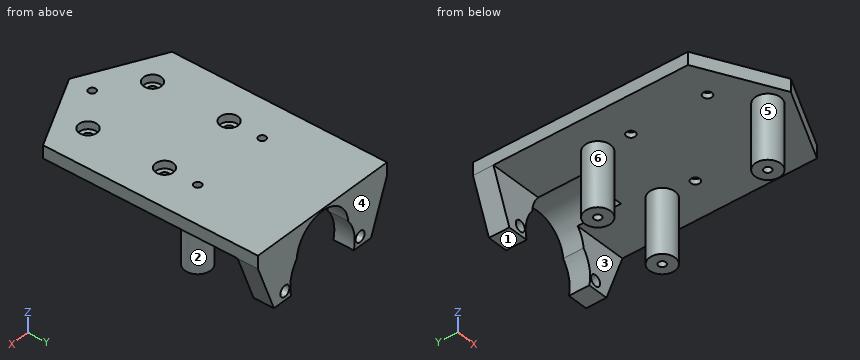
Autodesk Inventor part; units mm, degrees
ref_plane "YZ Plane" through (0, 0, 0) normal (1, 0, 0) x (0, 1, 0)
ref_plane "XZ Plane" through (0, 0, 0) normal (0, 1, 0) x (-1, 0, 0)
ref_plane "XY Plane" through (0, 0, 0) normal (0, 0, 1) x (1, 0, 0)
ref_plane "Work Plane1" through (0, 0, 0) normal (0, 0, 1) x (1, 0, 0)
sketch "Sketch1" plane through (0, 0, 0) normal (0, 0, 1) x (1, 0, 0)
  circle A0 centre (-15, -15) radius 1.5
  circle A1 centre (15, 15) radius 1.5
  circle A2 centre (15, -15) radius 1.5
  circle A3 centre (-15, 15) radius 1.5
  line L0 (30, 20) -> (-30, 20) construction
  line L1 (-30, 20) -> (-30, -20)
  line L2 (-30, -20) -> (30, -20)
  line L3 (30, -20) -> (30, 20)
  line L4 (30, 20) -> (-30, 20)
  line L5 (-30, 20) -> (-30, 64.25)
  line L6 (-30, 64.25) -> (30, 64.25)
  line L7 (30, 64.25) -> (30, 20)
  line L8 (13.5554, 64.25) -> (17.5, 64.25)
  line L9 (-30, -20) -> (0, -35)
  line L10 (0, -35) -> (30, -20)
  line L11 (-0.0001, -26) -> (-15, 28) construction
  line L12 (-15, 28) -> (15, 28) construction
  line L13 (15, 28) -> (-0.0001, -26) construction
  circle A4 centre (-15, 28) radius 1.45
  circle A5 centre (15, 28) radius 1.45
  circle A6 centre (0, -26.0002) radius 1.45
  line L14 (-30, -20) -> (30, -20)
  line L15 (30, -20) -> (30, 20)
  line L16 (30, 20) -> (-30, 20)
  line L17 (-30, 20) -> (-30, -20)
  point P0 (0, 0)
  dimension "d19" = 15
  dimension "d20" = 2.9
  dimension "d21" = 2.9
  dimension "d22" = 2.9
  dimension "d23" = 30
  dimension "d24" = 28
  dimension "d30" = 0
  dimension "d31" = 26
extrude "Extrusion1" add sketch "Sketch1" along normal blind 5 contours A0 | A1 | A2 | A3 | L4 L3 L2 L1 | L5 L6 L7 L4 | L2 L10 L9
sketch "Sketch2" plane through (0, 0, 5) normal (0, 0, 1) x (1, 0, 0)
  circle A0 centre (15, 15) radius 1.5
  circle A1 centre (15, -15) radius 1.5
  circle A2 centre (-20, 13) radius 1.5
  circle A3 centre (-20, -13) radius 1.5
  circle A4 centre (-15, -15) radius 1.5
  circle A5 centre (-15, 15) radius 1.5
  point P0 (0, 0)
hole "Hole1" at (15, 15, 5) at (15, -15, 5) at (-15, -15, 5) at (-15, 15, 5) direction (0, 0, -1) diameter 3.5 depth 8 tip angle 118 counterbore diameter 7 counterbore depth 3
sketch "Sketch3" plane through (-30, 64.25, 0) normal (0, 1, 0) x (1, 0, 0)
  circle A0 centre (12.5, 15.7367) radius 2.1
  circle A1 centre (47.5, 15.7367) radius 2.1
  arc A2 (16, 15.7367) -> (44, 15.7367) centre (30, 15.7367) ccw
  circle A3 centre (30, 15.7367) radius 15
  line L0 (12.5, 19.2367) -> (16.4446, 19.2367)
  line L1 (43.5554, 19.2367) -> (47.5, 19.2367)
  line L2 (15.414, 19.2367) -> (7.414, 19.2367)
  line L3 (0, 0) -> (60, 0)
  line L4 (7.414, 19.2367) -> (0, 0)
  line L5 (0, 0) -> (60, 0)
  line L6 (44.586, 19.2367) -> (52.586, 19.2367)
  line L7 (52.586, 19.2367) -> (60, 0)
  circle A4 centre (12.5, 15.7367) radius 1.45
  circle A5 centre (47.5, 15.7367) radius 1.45
  point P0 (30, 0)
  dimension "d9" = 30
  dimension "d10" = 8
  dimension "d11" = 8
  dimension "d12" = 2.9
  dimension "d13" = 2.9
extrude "Extrusion2" add sketch "Sketch3" against normal blind 8 contours A3 L1 L6 L7 L3 L4 L2 L0
sketch "Sketch4" plane through (-30, 64.25, 5) normal (0, 1, 0) x (1, 0, 0)
  circle A0 centre (30, 12.7367) radius 10
  circle A1 centre (30, 12.7367) radius 12
  point P0 (30, 5)
  dimension "d16" = 24
extrude "Extrusion3" cut sketch "Sketch4" against normal blind 25 contours A0 | A1
sketch "Sketch5" plane through (0, 0, 0) normal (0, 0, -1) x (-1, 0, 0)
  circle A0 centre (15, 15) radius 1.75
  circle A1 centre (-15, -15) radius 1.75
  circle A2 centre (-15, 15) radius 1.75
  circle A3 centre (15, -15) radius 1.75
  line L0 (9.173, 56.25) -> (9.173, 39.25)
  line L1 (9.173, 39.25) -> (-9.173, 39.25)
  line L2 (-9.173, 39.25) -> (-9.173, 56.25)
  line L3 (-9.173, 56.25) -> (-30, 56.25)
  line L4 (-30, -20) -> (-30, 56.25)
  line L5 (0, -35) -> (-30, -20)
  line L6 (30, -20) -> (0, -35)
  line L7 (30, 56.25) -> (9.173, 56.25)
  line L8 (30, -20) -> (30, 56.25)
  circle A4 centre (15, 28) radius 1.45
  circle A5 centre (-15, 28) radius 1.45
  circle A6 centre (0, -26.0002) radius 1.45
  circle A7 centre (15, 28) radius 1.45
  circle A8 centre (15, 28) radius 5
  circle A9 centre (-15, 28) radius 5
  circle A10 centre (0, -26.0002) radius 5
  point P0 (0, 0)
  dimension "d25" = 10
  dimension "d26" = 10
  dimension "d27" = 10
extrude "Extrusion4" add sketch "Sketch5" along normal blind 25 contours A8 | A9 | A10
properties part number "01_WG_writer_BASE"
Check sheet for the modelled part. Datum: model origin and axes. Units: mm. Face numbers are marked on the shaded views. A direction names the side the tool comes from. Round coordinates to 2 decimals unless told otherwise and drop trailing zeros. Order: outer loops, then holes, each group sorted by start corner. A loop starts at its lowest first (then second) coordinate and runs counter-clockwise, first axis right, second up. Notation, with made-up numbers: M -32.75,-5 L 2.25,-5 A12 ccw 2.25,8 Z; hole C 24,42 d5. An arc over 180 degrees is marked long. One line per item, written item: value. Start each with the question number.
1. Section check B-B on y = 15. Enter the section's corners in (x, z).
2. Section check C-C on x = 21. Enter the section's corners in (y, z), and give its area (3 significant figures).
3. Scan lines: line 1 along Y through (x, z) = (-15, -18); line 2 along X through (y, z) = (-15, 1.25); line 3 along X through (y, z) = (58, -15.5). Record each from-to range of solid material in increasing order.
4. Access from +Z, -Z, +X, -X, +Y, -Y to the whole of each face (thin tool, end or side, straight path). Record for the marked faces 1, 2 and 3.
5. Gauge pin test, flat ends, axial feed: P1, Ø6.5, axis at x = 18.5, y = 60.5, coming from the -Z side; P2, Ø2, axis at x = -22.5, y = -10.5, coming from the -Z side; P3, Ø9, axis at x = -15, y = 15, coming from the +Z side; P4, Ø1.5, axis at y = -24, z = -21, coming from the -X side. Record the tip position at first contact, or that the pin passes through.
6. Section check A-A on z = -3. Enter the section's corners in (x, y).
7. Release check for a two-part mould opening along X. For the marked faces 4, 5 and 6 record: released by +X, released by -X, zero draft, split by the parting line, or undercut.
8. Section check D-D on z = -16.75. Give the number of separate pieces and of enclosed holes in the cut face, and give its area (3 significant figures).
Results found:
1. outline: M -30,0 L -16.75,0 L -16.75,2 L -18.5,2 L -18.5,5 L -30,5 Z; M -13.25,0 L 13.25,0 L 13.25,2 L 11.5,2 L 11.5,5 L -11.5,5 L -11.5,2 L -13.25,2 Z; M 16.75,0 L 30,0 L 30,5 L 18.5,5 L 18.5,2 L 16.75,2 Z
2. outline: M -24.5,0 L 56.25,0 L 56.25,-19.24 L 64.25,-19.24 L 64.25,5 L -24.5,5 Z
2. area: 598 mm^2
3. line 1: 23 to 26.55, 29.45 to 33, 56.25 to 64.25
3. line 2: -30 to -16.75, -13.25 to 13.25, 16.75 to 30
3. line 3: -24.03 to -19.59, -15.41 to -15, 15 to 15.41, 19.59 to 24.03
4. face 1: -Z, +X, -X, +Y
4. face 2: -Z
4. face 3: -Z, +X, -X
5. P1: z = -19.24
5. P2: z = 0
5. P3: z = 5
5. P4: x = -4.84
6. outline: M -28.84,56.25 L -11.03,56.25 L -11.03,64.25 L -28.84,64.25 Z; C -15,28 d10; C 0,-26 d10; C 15,28 d10; M 11.03,56.25 L 28.84,56.25 L 28.84,64.25 L 11.03,64.25 Z; hole C -15,28 d2.9; hole C 0,-26 d2.9; hole C 15,28 d2.9
7. face 4: zero draft
7. face 5: split by the parting line
7. face 6: undercut
8. separate pieces: 7
8. enclosed holes: 3
8. area: 294 mm^2
